```python
from build123d import *

# Parameters (mm, degrees)
SKETCH1_R           = 1.5
BOSS_EXTRUDE1_DEPTH = 55
SKETCH2_W           = 3.168024794
SKETCH2_H           = 0.5


with BuildPart() as part:
    # Sketch1 → Boss-Extrude1 (new body)
    with BuildSketch(Plane.XY):
        Circle(SKETCH1_R)
    extrude(amount=BOSS_EXTRUDE1_DEPTH)

    # Sketch2 → Cut-Revolve1 (revolve, cut)
    with BuildSketch(Plane(origin=(0, 0, 0), x_dir=(1, 0, 0), z_dir=(0, 1, 0))):
        with Locations((-2.784012397, -1.25)):
            Rectangle(SKETCH2_W, SKETCH2_H)
    cut_revolve1 = revolve(axis=Axis((0, 0, 0), (0, 0, 1)), mode=Mode.SUBTRACT)

    # Mirror1: Cut-Revolve1 across plane
    add(cut_revolve1.mirror(Plane.XY.offset(27.5)), mode=Mode.SUBTRACT)


solid = part.part
```
Part model, mm, in its own coordinate system. A direction names the side the tool comes from. Round coordinates to 2 decimals unless told otherwise and drop trailing zeros. Write each loop counter-clockwise with the first axis right and the second up, starting at its lowest first coordinate (ties: lowest second). Pieces come first, ordered by that corner, then holes. Notation, with made-up numbers: (23.5, 18.5) -> (80.5, 18.5) arc R12 cw to (80.5, 32.5) -> close; hole circle Ø1 at (28, 74.25). An arc over 180 degrees is marked (long way). Return JSON: item names as keys, results as strings. Group by question number.
Q1. Saw through at B-B on z = 31.5. Write the cut outline in (x, y), plus the area to 3 significant figures.
Q2. Mould opens along Z. For faces 1 (the cylindrical face through (-1.5, 0.07, 54.49)), 2 (the cylindrical face through (-0.65, -1.01, 1.25)), 3 (the flat face through (0, 0, 55)) say: pulls with the +Z half, pulls with the -Z half, needs draft (parallel to the pull), parting line crosses it, or undercut.
Q3. Saw through at A-A on x = -0.65. Write the cut outline in (y, z).
Q4. Which spindle directions (+Z, -Z, +X, -X, +Y, -Y) get a long thin tool onto all of the face, cutting with end or side? Do faces 4 (the cylindrical face through (-1.5, 0.07, 27.14)), 5 (the cylindrical face through (-0.65, -1.01, 53.75)). Say none if no direction does.
Q5. Probe L1, parallel to Z at x = -0.6, y = -1.3; L2, parallel to Y at x = -0.9, z = 27; L3, parallel to X at y = 0.15, z = 16. List the from-to ranges inside material, lowest first. Write a range as [from, to].
Answer:
{
 "1": {"outline": "circle Ø3 at (0, 0)", "area": "7.07 mm2"},
 "2": {"face 1": "needs draft", "face 2": "undercut", "face 3": "pulls with the +Z half"},
 "3": {"outline": "(-1.35, 0) -> (1.35, 0) -> (1.35, 1) -> (1.01, 1) -> (1.01, 1.5) -> (1.35, 1.5) -> (1.35, 53.5) -> (1.01, 53.5) -> (1.01, 54) -> (1.35, 54) -> (1.35, 55) -> (-1.35, 55) -> (-1.35, 54) -> (-1.01, 54) -> (-1.01, 53.5) -> (-1.35, 53.5) -> (-1.35, 1.5) -> (-1.01, 1.5) -> (-1.01, 1) -> (-1.35, 1) -> close"},
 "4": {"face 4": "+Z, -Z", "face 5": "none"},
 "5": {"L1": "[0, 1], [1.5, 53.5], [54, 55]", "L2": "[-1.2, 1.2]", "L3": "[-1.49, 1.49]"}
}
